Build history of the part. All positions in model axes, mm. Coordinates: 2 decimals unless noted, no trailing zeros. Order: outer loops, then holes, each group sorted by start corner. A loop starts at its lowest first (then second) coordinate and runs counter-clockwise, first axis right, second up. Notation, with made-up numbers: (84, 47) - (117, 47) arc R17 cw to (117, 55) - close; hole circle Ø8 at (59.25, -25). An arc over 180 degrees is marked (long way). Write each question's results on one line, items separated by ' | '.
from build123d import *

# Parameters (mm, degrees)
SKETCH1_R           = 1.6
BOSS_EXTRUDE1_DEPTH = 3
SKETCH2_R           = 1.6
CUT_EXTRUDE1_DEPTH  = 45
SKETCH3_R           = 1.6
CUT_EXTRUDE2_DEPTH  = 89.509886453


with BuildPart() as part:
    # Sketch1 → Boss-Extrude1 (new body)
    with BuildSketch(Plane(origin=(0, 0, 0), x_dir=(1, 0, 0), z_dir=(0, 1, 0))):
        with BuildLine():
            Line((-50, 65), (50, 65))
            ThreePointArc((50, 65), (57.071067812, 62.071067812), (60, 55))
            Line((60, 55), (60, -55))
            ThreePointArc((60, -55), (57.071067812, -62.071067812), (50, -65))
            Line((50, -65), (-50, -65))
            ThreePointArc((-50, -65), (-57.071067812, -62.071067812), (-60, -55))
            Line((-60, -55), (-60, 55))
            ThreePointArc((-60, 55), (-57.071067812, 62.071067812), (-50, 65))
        make_face()
        with Locations(Location((50, -55, 0), (0, 0, 90))):
            Circle(SKETCH1_R, mode=Mode.SUBTRACT)
        with Locations(Location((50, 55, 0), (0, 0, 270))):
            Circle(SKETCH1_R, mode=Mode.SUBTRACT)
        with Locations(Location((-50, -55, 0), (0, 0, 270))):
            Circle(SKETCH1_R, mode=Mode.SUBTRACT)
        with Locations(Location((-50, 55, 0), (0, 0, 90))):
            Circle(SKETCH1_R, mode=Mode.SUBTRACT)
        with BuildLine():
            Line((-15, -42.267985155), (15, -42.267985155))
            ThreePointArc((15, -42.267985155), (21, -48.267985155), (15, -54.267985155))
            Line((15, -54.267985155), (-15, -54.267985155))
            ThreePointArc((-15, -54.267985155), (-21, -48.267985155), (-15, -42.267985155))
        make_face(mode=Mode.SUBTRACT)
    extrude(amount=BOSS_EXTRUDE1_DEPTH)

    # Sketch2 → Cut-Extrude1 (cut)
    with BuildSketch(Plane(origin=(0, 0, 0), x_dir=(1, 0, 0), z_dir=(0, 1, 0))):
        with Locations(Location((29, 30.5, 0), (0, 0, 90))):
            Circle(SKETCH2_R)
        with Locations(Location((-29, 30.5, 0), (0, 0, 90))):
            Circle(SKETCH2_R)
        with Locations(Location((29, -30.5, 0), (0, 0, 90))):
            Circle(SKETCH2_R)
        with Locations(Location((-29, -30.5, 0), (0, 0, 90))):
            Circle(SKETCH2_R)
    extrude(amount=CUT_EXTRUDE1_DEPTH, mode=Mode.SUBTRACT)

    # Sketch3 → Cut-Extrude2 (cut, through all)
    with BuildSketch(Plane(origin=(0, 3, 0), x_dir=(1, 0, 0), z_dir=(0, 1, 0))):
        with Locations(Location((-15, 55, 0), (0, 0, 270))):
            Circle(SKETCH3_R)
        with Locations(Location((15, 55, 0), (0, 0, 270))):
            Circle(SKETCH3_R)
    extrude(amount=-CUT_EXTRUDE2_DEPTH, mode=Mode.SUBTRACT)


solid = part.part
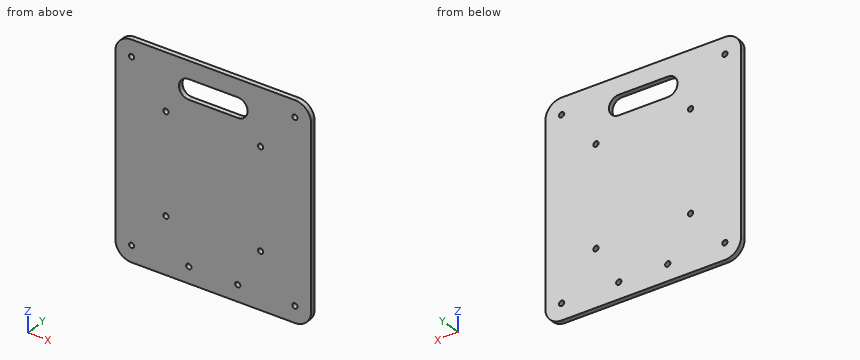
1. Band-saw the part on A-A on z = 30.5. Give the cut face in (x, y), then the cut area to 3 significant figures.
Solved:
outline: (-60, 0) - (-30.6, 0) - (-30.6, 3) - (-60, 3) - close; (-27.4, 0) - (27.4, 0) - (27.4, 3) - (-27.4, 3) - close; (30.6, 0) - (60, 0) - (60, 3) - (30.6, 3) - close | area: 341 mm2
2. Band-saw the part on C-C on z = 46. Give the cut face in (x, y).
Solved:
outline: (-60, 0) - (-20.55, 0) - (-20.55, 3) - (-60, 3) - close; (20.55, 0) - (60, 0) - (60, 3) - (20.55, 3) - close
3. Drop flat-ended pins along their axis: pin 1 Ø3.5 at (x, z) = (50, -55) entering from +Y; pin 2 Ø1.9 at (x, z) = (50, 55) entering from -Y. Give the stop position or say it passes through.
Solved:
pin 1: stops at y = 3 | pin 2: passes through
4. Probe line 1 (X direction, y = 1.4, z = 55); line 2 (X direction, y = 0.9, z = 30.5); line 3 (Z direction, x = -29, y = 1.3). List the from-to ranges inside material, lowest first.
Solved:
line 1: x = -60 to -51.6, -48.4 to 48.4, 51.6 to 60 | line 2: x = -60 to -30.6, -27.4 to 27.4, 30.6 to 60 | line 3: z = -65 to -32.1, -28.9 to 28.9, 32.1 to 65
5. Band-saw the part on B-B on y = 2. Give the number of separate pieces and of enclosed holes in the cut face, then the cut area to 3 significant figures.
Solved:
separate pieces: 1 | enclosed holes: 11 | area: 15,000 mm2
